Build history of the part. All positions in model axes, mm. A direction names the side the tool comes from. Round coordinates to 2 decimals unless told otherwise and drop trailing zeros. Write each loop counter-clockwise with the first axis right and the second up, starting at its lowest first coordinate (ties: lowest second). Pieces come first, ordered by that corner, then holes.
from build123d import *

# Parameters (mm, degrees)
SKETCH1_W           = 25.4
SKETCH1_H           = 25.4
SKETCH1_W_2         = 19.05
SKETCH1_H_2         = 19.05
BOSS_EXTRUDE1_DEPTH = 508
SKETCH2_R           = 3.175
CUT_EXTRUDE1_DEPTH  = 510.268416456
CUT_EXTRUDE2_REACH  = 511.268
SKETCH3_R           = 2.5796875


with BuildPart() as part:
    # Sketch1 → Boss-Extrude1 (new body)
    with BuildSketch(Plane(origin=(0, 0, 0), x_dir=(1, 0, 0), z_dir=(0, 1, 0))):
        with Locations((12.7, 12.7)):
            Rectangle(SKETCH1_W, SKETCH1_H)
        with Locations((12.7, 12.7)):
            Rectangle(SKETCH1_W_2, SKETCH1_H_2, mode=Mode.SUBTRACT)
    extrude(amount=BOSS_EXTRUDE1_DEPTH)

    # Sketch2 → Cut-Extrude1 (cut, through all)
    with BuildSketch(Plane(origin=(25.4, 0, 0), x_dir=(0, 0, -1), z_dir=(1, 0, 0))):
        with Locations((12.7, 12.7)):
            Circle(SKETCH2_R)
    cut_extrude1 = extrude(amount=-CUT_EXTRUDE1_DEPTH, mode=Mode.SUBTRACT)

    # Mirror1: Cut-Extrude1 across plane
    add(cut_extrude1.mirror(Plane.ZX.offset(254)), mode=Mode.SUBTRACT)

    # Sketch3 → Cut-Extrude2 (cut, up to next)
    with BuildSketch(Plane(origin=(25.4, 0, 0), x_dir=(0, 0, -1), z_dir=(1, 0, 0)), mode=Mode.PRIVATE) as cut_extrude2_sk1:
        with Locations((12.7, 304.800000001)):
            Circle(SKETCH3_R)
    cut_extrude2_tool1 = extrude(cut_extrude2_sk1.sketch, amount=-CUT_EXTRUDE2_REACH, mode=Mode.PRIVATE) & part.part
    # Sketch3 → Cut-Extrude2 (cut, up to next)
    with BuildSketch(Plane(origin=(25.4, 0, 0), x_dir=(0, 0, -1), z_dir=(1, 0, 0)), mode=Mode.PRIVATE) as cut_extrude2_sk2:
        with Locations((12.7, 355.600000001)):
            Circle(SKETCH3_R)
    cut_extrude2_tool2 = extrude(cut_extrude2_sk2.sketch, amount=-CUT_EXTRUDE2_REACH, mode=Mode.PRIVATE) & part.part
    # Sketch3 → Cut-Extrude2 (cut, up to next)
    with BuildSketch(Plane(origin=(25.4, 0, 0), x_dir=(0, 0, -1), z_dir=(1, 0, 0)), mode=Mode.PRIVATE) as cut_extrude2_sk3:
        with Locations((12.7, 203.200000001)):
            Circle(SKETCH3_R)
    cut_extrude2_tool3 = extrude(cut_extrude2_sk3.sketch, amount=-CUT_EXTRUDE2_REACH, mode=Mode.PRIVATE) & part.part
    # Sketch3 → Cut-Extrude2 (cut, up to next)
    with BuildSketch(Plane(origin=(25.4, 0, 0), x_dir=(0, 0, -1), z_dir=(1, 0, 0)), mode=Mode.PRIVATE) as cut_extrude2_sk4:
        with Locations((12.7, 152.400000001)):
            Circle(SKETCH3_R)
    cut_extrude2_tool4 = extrude(cut_extrude2_sk4.sketch, amount=-CUT_EXTRUDE2_REACH, mode=Mode.PRIVATE) & part.part
    add(cut_extrude2_tool1.solids().sort_by_distance((25.4, 304.8, -12.7))[0], mode=Mode.SUBTRACT)
    add(cut_extrude2_tool2.solids().sort_by_distance((25.4, 355.6, -12.7))[0], mode=Mode.SUBTRACT)
    add(cut_extrude2_tool3.solids().sort_by_distance((25.4, 203.2, -12.7))[0], mode=Mode.SUBTRACT)
    add(cut_extrude2_tool4.solids().sort_by_distance((25.4, 152.4, -12.7))[0], mode=Mode.SUBTRACT)


solid = part.part
1) Pin check, flat tips, straight feed: pin 1 Ø10 at (y, z) = (12.7, -12.7) entering from -X; pin 2 Ø4.5 at (y, z) = (203.2, -12.7) entering from +X (3 decimals). Stop position of each tip, or through.
Results:
pin 1: stops at x = 0
pin 2: stops at x = 3.175
2) Slice it at B-B (y = 189.5). Write the cut outline in (x, z) (3 decimals), plus the area to 3 significant figures.
Results:
outline: (0, -25.4) - (25.4, -25.4) - (25.4, 0) - (0, 0) - close; hole (3.175, -22.225) - (22.225, -22.225) - (22.225, -3.175) - (3.175, -3.175) - close
area: 282 mm2
3) Mould opens along X. For faces 1 (the flat face through (0, 250, -13)), 2 (the flat face through (22.225, 250, -13)), 3 (the flat face through (24, 508, -13)), 4 (the flat face through (3.175, 250, -13)) say: released by +X, released by -X, zero draft, split by the parting line, or undercut.
Results:
face 1: released by -X
face 2: undercut
face 3: zero draft
face 4: undercut
4) Wall check: L1, parallel to X at y = 63.5, z = -3.25 (3 decimals); L2, parallel to Z at x = 7.75, y = 486 (3 decimals); L3, parallel to Z at x = 0.7, y = 495.3 (3 decimals). Give the ranges that are in metal, low to high.
Results:
L1: x = 0 to 3.175, 22.225 to 25.4
L2: z = -25.4 to -22.225, -3.175 to 0
L3: z = -25.4 to -15.875, -9.525 to 0
5) Slice it at A-A (x = 9). Write the cut outline in (y, z) (3 decimals).
Results:
outline: (0, -25.4) - (508, -25.4) - (508, -22.225) - (0, -22.225) - close; (0, -3.175) - (508, -3.175) - (508, 0) - (0, 0) - close
6) Which spindle directions (+Z, -Z, +X, -X, +Y, -Y) get a long thin tool onto all of the face, cutting with end or side? Do faces 5 (the flat face through (13, 250, 0)), 6 (the flat face through (13, 250, -22.225)). Say none if no direction does.
Results:
face 5: +Z, +X, -X, +Y, -Y
face 6: +Y, -Y
